from build123d import *

# Parameters (mm, degrees)
F0_R      = 6.65
F0_R_2    = 0.889
F1_DEPTH  = 12.7
F2_R      = 1.075
F3_DEPTH  = 9.525
F4_R      = 6.35
F5_R      = 6.35
F6_R      = 6.35
F12_R     = 6.15
F14_R     = 0.889
F15_DEPTH = 15.1883232269
F16_R     = 0.889
F17_DEPTH = 25.1606906232


with BuildPart() as f1:
    # F0 (on Right) → F1 (new body)
    with BuildSketch(Plane.YZ):
        Polygon((0, 76.2), (-50.8, 76.2), (-50.8, -50.8), (101.6, -50.8), (101.6, 0), (0, 0), align=None)
        with Locations((-19.05, -25.4)):
            Circle(F0_R, mode=Mode.SUBTRACT)
        with Locations((22.4592145532, -36.9)):
            Circle(F0_R_2, mode=Mode.SUBTRACT)
        with Locations((22.4592145532, -13.9)):
            Circle(F0_R_2, mode=Mode.SUBTRACT)
        with Locations((80.4592145532, -36.9)):
            Circle(F0_R_2, mode=Mode.SUBTRACT)
        with Locations((80.4592145532, -13.9)):
            Circle(F0_R_2, mode=Mode.SUBTRACT)
    extrude(amount=F1_DEPTH)

    # F2 (on face) → F3 (join)
    with BuildSketch(Plane.YZ.offset(12.7)):
        with Locations((-31.0889787972, -14.9)):
            Circle(F2_R)
        with Locations((-18.5889787972, -14.9)):
            Circle(F2_R)
        with Locations((-18.5889787972, -35.9)):
            Circle(F2_R)
        with Locations((-31.0889787972, -35.9)):
            Circle(F2_R)
    extrude(amount=F3_DEPTH)

    # F4
    f4_edges = [f1.edges().sort_by_distance(p)[0] for p in [
        (6.35, 0, 0),
    ]]
    fillet(f4_edges, radius=F4_R)

    # F5
    f5_edges = [f1.edges().sort_by_distance(p)[0] for p in [
        (6.35, -50.8, -50.8),
        (6.35, -50.8, 76.2),
        (6.35, 101.6, -50.8),
    ]]
    fillet(f5_edges, radius=F5_R)

    # F6
    f6_edges = [f1.edges().sort_by_distance(p)[0] for p in [
        (6.35, 0, 76.2),
        (6.35, 101.6, 0),
    ]]
    fillet(f6_edges, radius=F6_R)

    # F13: sweep along a path in F9
    with BuildLine(Plane(origin=(0, -19.05, 0), x_dir=(-1, 0, 0), z_dir=(0, 1, 0))) as f13_path:
        Line((69.4630440448, 35.1738945205), (-53.2095358939, 68.0439132485))
    # F12 (on plane+point) → F13 (sweep, cut)
    with BuildSketch(Plane(origin=(66.6561511629, 0, 17.8604618747), x_dir=(0, 1, 0), z_dir=(0.9659258263, 0, 0.2588190451))):
        with Locations((-19.05, 51.9537318581)):
            Circle(F12_R)
    sweep(path=f13_path.line, mode=Mode.SUBTRACT)

    # F14 (on face) → F15 (cut, through all)
    with BuildSketch(Plane.XY.offset(76.2)):
        with Locations((4.0958291739, -19.05)):
            Circle(F14_R)
    extrude(amount=-F15_DEPTH, mode=Mode.SUBTRACT)

    # F16 (on face) → F17 (cut, through all)
    with BuildSketch(Plane.XZ.offset(50.8)):
        with Locations((6.35, -25.4)):
            Circle(F16_R)
    extrude(amount=-F17_DEPTH, mode=Mode.SUBTRACT)


solid = f1.part
The model under review builds one solid part; all positions refer to its coordinate system, in mm. A direction names the side the tool comes from. Coordinates: 2 decimals unless noted, no trailing zeros. Loops run counter-clockwise (first coordinate to the right, second up) from the corner with the lowest first, then second, coordinate; pieces in that order, holes last. Notation, with made-up numbers: (15.25, -7) -> (45.25, -7) arc R20 cw to (45.25, 16) -> close; hole circle Ø3 at (-7.75, -35.75). An arc over 180 degrees is marked (long way). Use a Markdown table: item, result. Add a question column.
1. Add section B-B on x = 14.75. Write out the cut boundary in (y, z) (3 decimals).
2. To check wall thickness, follow line 1 (Z direction, x = 6.35, y = -38.5); line 2 (Y direction, x = 9.5, z = -36.9); line 3 (Y direction, x = 20, z = -36). State the ranges of each line that lie inside material, in increasing order.
3. Clearance check with flat-ended pins moving along their axes: pin 1 Ø5 at (x, z) = (3, 61) entering from +Y; pin 2 Ø2 at (x, z) = (6.35, -25.4) entering from -Y; pin 3 Ø1.4 at (x, y) = (4.1, -19.05) entering from +Z; pin 4 Ø4 at (x, y) = (4, 35) entering from +Z. State where each tip first meets the part, or that it passes through.
4. Draft analysis for pull direction Y (two halves, no side actions). For faces 1 (the face through (6.44, -1.91, 74.39)), 2 (the face through (6.44, -48.89, 74.39)), 3 (the face through (6.26, -12.91, -27.95)), state which applies: pulls with the +Y half, pulls with the -Y half, needs draft (parallel to the pull), parting line crosses it, or undercut.
5. Add section A-A on y = -41. Write out the cut boundary in (x, z).
6. Add section C-C on z = 30. Write out the cut boundary in (x, y), plus the area to 3 significant figures.
7. Machinability: for faces 4 (the face through (6, 0, 38)), 5 (the face through (0, 7, -1)), which of the approach directions +Z, -Z, +X, -X, +Y, -Y give a long, thin tool a straight path to every point of the face, cutting with its end or side? Answer none if there is none.
Returned:
| question | item | result |
|---|---|---|
| 1 | outline | circle Ø2.15 at (-31.089, -35.9); circle Ø2.15 at (-31.089, -14.9); circle Ø2.15 at (-18.589, -35.9); circle Ø2.15 at (-18.589, -14.9) |
| 2 | line 1 | z = -50.8 to -26.29, -24.51 to 76.2 |
| 2 | line 2 | y = -50.8 to 21.57, 23.35 to 79.57, 81.35 to 101.6 |
| 2 | line 3 | y = -32.16 to -30.02, -19.66 to -17.52 |
| 3 | pin 1 | stops at y = 0 |
| 3 | pin 2 | stops at y = -50.8 |
| 3 | pin 3 | stops at z = 48.71 |
| 3 | pin 4 | stops at z = 0 |
| 4 | face 1 | pulls with the +Y half |
| 4 | face 2 | pulls with the -Y half |
| 4 | face 3 | undercut |
| 5 | outline | (0, -50.8) -> (12.7, -50.8) -> (12.7, 76.2) -> (0, 76.2) -> close; hole circle Ø1.78 at (6.35, -25.4) |
| 6 | outline | (0, -50.8) -> (12.7, -50.8) -> (12.7, 0) -> (0, 0) -> close |
| 6 | area | 645 mm² |
| 7 | face 4 | +Z, +X, -X, +Y |
| 7 | face 5 | +Z, -Z, -X, +Y, -Y |
